from build123d import *

# Parameters (mm, degrees)
BOSS_EXTRUDE1_DEPTH = 6.73
CUT_EXTRUDE5_DEPTH  = 6.73
SKETCH4_R           = 7.35
BOSS_EXTRUDE2_DEPTH = 21.59
SKETCH5_R           = 6.35
CUT_EXTRUDE6_DEPTH  = 46.540850343
BOSS_EXTRUDE3_START = -10
SKETCH6_R           = 8.466621056
SKETCH6_R_2         = 7.35
BOSS_EXTRUDE3_DEPTH = 10
SKETCH7_R           = 2.5
SKETCH7_R_2         = 2.34
BOSS_EXTRUDE4_DEPTH = 6.73


with BuildPart() as part:
    # Sketch1 → Boss-Extrude1 (new body)
    with BuildSketch(Plane(origin=(0, 0, 0), x_dir=(0, 0, -1), z_dir=(1, 0, 0))):
        with BuildLine():
            Line((14.28, 0), (2.5, 0))
            ThreePointArc((2.5, 0), (0, -2.5), (-2.5, 0))
            Line((-2.5, 0), (-4.795, 0))
            Line((-4.795, 0), (-4.795, -12.615))
            Line((-4.795, -12.615), (14.28, -12.615))
            Line((14.28, -12.615), (14.28, 0))
        make_face()
        with BuildLine():
            ThreePointArc((-2.5, 0), (0, 2.5), (2.5, 0))
            Line((2.5, 0), (14.28, 0))
            Line((14.28, 0), (14.28, 12.625))
            Line((14.28, 12.625), (-4.795, 12.625))
            Line((-4.795, 12.625), (-4.795, 0))
            Line((-4.795, 0), (-2.5, 0))
        make_face()
        with BuildLine():
            Line((14.28, 12.625), (14.28, 0))
            Line((14.28, 0), (26.06, 0))
            ThreePointArc((26.06, 0), (28.56, 2.5), (31.06, 0))
            Line((31.06, 0), (33.355, 0))
            Line((33.355, 0), (33.355, 12.625))
            Line((33.355, 12.625), (14.28, 12.625))
        make_face()
        with BuildLine():
            Line((26.06, 0), (14.28, 0))
            Line((14.28, 0), (14.28, -12.615))
            Line((14.28, -12.615), (33.355, -12.615))
            Line((33.355, -12.615), (33.355, 0))
            Line((33.355, 0), (31.06, 0))
            ThreePointArc((31.06, 0), (28.56, -2.5), (26.06, 0))
        make_face()
    extrude(amount=BOSS_EXTRUDE1_DEPTH)

    # Sketch3 → Cut-Extrude5 (cut)
    with BuildSketch(Plane.ZY):
        with BuildLine():
            Line((4.795, -12.615), (4.795, 0))
            ThreePointArc((4.795, 0), (4.113307599, -6.450002601), (2.098352225, -12.615))
            Line((2.098352225, -12.615), (4.795, -12.615))
        make_face()
        with BuildLine():
            Line((4.795, 12.625), (2.093870071, 12.625))
            ThreePointArc((2.093870071, 12.625), (4.112161723, 6.455360716), (4.795, 0))
            Line((4.795, 0), (4.795, 12.625))
        make_face()
        with BuildLine():
            ThreePointArc((-33.355, 1.23e-07), (-32.67216171, 6.455360776), (-30.653870071, 12.625))
            Line((-30.653870071, 12.625), (-33.355, 12.625))
            Line((-33.355, 12.625), (-33.355, 1.23e-07))
        make_face()
        with BuildLine():
            ThreePointArc((-30.658352225, -12.615), (-32.673307611, -6.450002541), (-33.355, 1.23e-07))
            Line((-33.355, 1.23e-07), (-33.355, -12.615))
            Line((-33.355, -12.615), (-30.658352225, -12.615))
        make_face()
    extrude(amount=-CUT_EXTRUDE5_DEPTH, mode=Mode.SUBTRACT)

    # Sketch4 → Boss-Extrude2 (add)
    with BuildSketch(Plane.ZY):
        with Locations(Location((-14.28, 0, 0), (0, 0, 180))):
            Circle(SKETCH4_R)
    extrude(amount=BOSS_EXTRUDE2_DEPTH)

    # Sketch5 → Cut-Extrude6 (cut, through all)
    with BuildSketch(Plane.ZY.offset(21.59)):
        with Locations((-14.28, 0)):
            Circle(SKETCH5_R)
    extrude(amount=-CUT_EXTRUDE6_DEPTH, mode=Mode.SUBTRACT)

    # Sketch6 → Boss-Extrude3 (add)
    with BuildSketch(Plane.ZY.offset(21.59).offset(BOSS_EXTRUDE3_START)):
        with Locations((-14.28, 0)):
            Circle(SKETCH6_R)
        with Locations(Location((-14.28, 0, 0), (0, 0, 180))):
            Circle(SKETCH6_R_2, mode=Mode.SUBTRACT)
    extrude(amount=BOSS_EXTRUDE3_DEPTH)

    # Sketch7 → Boss-Extrude4 (add, through all)
    # profile 1 of 2: a face of its own
    with BuildSketch(Plane.ZY):
        with Locations((-28.56, 0)):
            Circle(SKETCH7_R)
        with Locations((-28.56, 0)):
            Circle(SKETCH7_R_2, mode=Mode.SUBTRACT)
    # profile 2 of 2: a face of its own
    with BuildSketch(Plane.ZY):
        Circle(SKETCH7_R)
        Circle(SKETCH7_R_2, mode=Mode.SUBTRACT)
    extrude(amount=-BOSS_EXTRUDE4_DEPTH)


solid = part.part
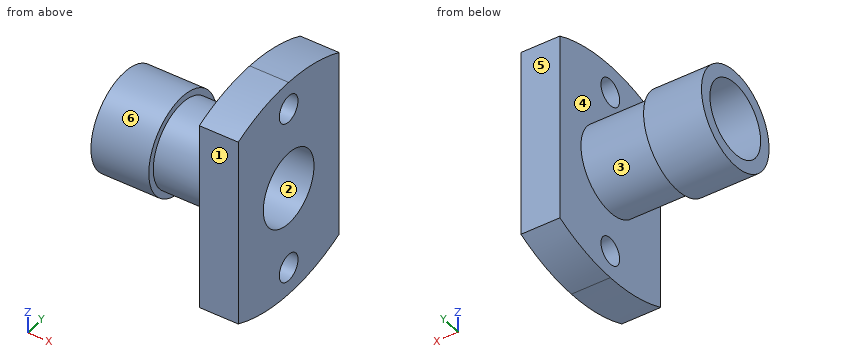
The model under review builds one solid part; all positions refer to its coordinate system, in mm. Face numbers are marked on the shaded views. A direction names the side the tool comes from. Give positions to 0.01 mm unless a question says otherwise; leave off trailing zeros. Loops run counter-clockwise (first coordinate to the right, second up) from the corner with the lowest first, then second, coordinate; pieces in that order, holes last. Notation, with made-up numbers: (67.5, 82.25) -> (75.5, 82.25) arc R36 cw to (75.5, 120.25) -> close; hole circle Ø3 at (3.25, -24.75). An arc over 180 degrees is marked (long way). Answer as a JSON object with one key per item and string values. Group by question number.
Q1. Wall thickness on line 1 along Y through (x, z) = (-5.5, -14.28); line 2 along X through (y, z) = (-7.5, -14); line 3 along Y through (x, z) = (2, -28.56) (3 decimals): over which ranges is each line inside the solid? List them lowest first.
Q2. Insertion check: pin 1 (8 mm diameter, centred on y = 9, z = -1, fed in from -X); pin 2 (1.5 mm diameter, centred on x = 1.5, y = 1.5, fed in from -Z); pin 3 (5 mm diameter, centred on y = 3, z = -17.5, fed in from +X); pin 4 (10 mm diameter, centred on x = -2.5, y = 5, fed in from +Z). Each pin has a flat end and moves straight along its axis. Give the tip position at first contact, or say it passes through.
Q3. Take a section at D-D (z = -14.28). Write out the cut boundary in (x, y) (3 decimals).
Q4. Take a section at A-A (z = 0). Write out the cut boundary in (x, y) (3 decimals), plus the area to 3 significant figures.
Q5. Draft analysis for pull direction Y (two halves, no side actions). For the marked faces 1, 2, 3 and 4, state which applies: pulls with the +Y half, pulls with the -Y half, needs draft (parallel to the pull), parting line crosses it, or undercut.
Q6. Tool access review of the marked faces 5 and 6: name each direction out of +Z, -Z, +X, -X, +Y, -Y from which nothing blocks a thin tool from reaching the whole face with its end or side.
Q7. Take a section at B-B (y = -4.25). Write out the cut boundary in (x, z), plus the area to 3 significant figures.
Q8. Take a section at C-C (x = 2). Write out the cut boundary in (y, z) (3 decimals).
Answer below:
{
 "1": {"line 1": "y = -7.35 to -6.35, 6.35 to 7.35", "line 2": "x = -21.59 to -11.59, 0 to 6.73", "line 3": "y = -12.615 to -2.34, 2.34 to 12.625"},
 "2": {"pin 1": "stops at x = 0", "pin 2": "stops at z = -33.35", "pin 3": "stops at x = 6.73", "pin 4": "stops at z = 4.79"},
 "3": {"outline": "(-21.59, -8.467) -> (-11.59, -8.467) -> (-11.59, -7.35) -> (0, -7.35) -> (0, -12.615) -> (6.73, -12.615) -> (6.73, -6.35) -> (-21.59, -6.35) -> close; (-21.59, 6.35) -> (6.73, 6.35) -> (6.73, 12.625) -> (0, 12.625) -> (0, 7.35) -> (-11.59, 7.35) -> (-11.59, 8.467) -> (-21.59, 8.467) -> close"},
 "4": {"outline": "(0, -12.615) -> (6.73, -12.615) -> (6.73, -2.34) -> (0, -2.34) -> close; (0, 2.34) -> (6.73, 2.34) -> (6.73, 12.625) -> (0, 12.625) -> close", "area": "138 mm2"},
 "5": {"face 1": "pulls with the -Y half", "face 2": "undercut", "face 3": "parting line crosses it", "face 4": "needs draft"},
 "6": {"face 5": "+Z, -Z, +X, -X, +Y", "face 6": "-X"},
 "7": {"outline": "(-21.59, -21.6) -> (-11.59, -21.6) -> (-11.59, -20.28) -> (0, -20.28) -> (0, -33.06) -> (6.73, -33.06) -> (6.73, -19) -> (-21.59, -19) -> close; (-21.59, -9.56) -> (6.73, -9.56) -> (6.73, 4.5) -> (0, 4.5) -> (0, -8.28) -> (-11.59, -8.28) -> (-11.59, -6.96) -> (-21.59, -6.96) -> close", "area": "271 mm2"},
 "8": {"outline": "(-12.615, -30.658) arc R30.855 ccw to (12.625, -30.654) -> (12.625, 2.094) arc R30.855 ccw to (-12.615, 2.098) -> close; hole circle Ø12.7 at (0, -14.28); hole circle Ø4.68 at (0, -28.56); hole circle Ø4.68 at (0, 0)"}
}
